from build123d import *

# Parameters (mm, degrees)
F1_DEPTH = 19.05
F2_R     = 88.9
F3_R     = 12.69999
F5_DEPTH = 19.051


# Not quite as in the source:
# - a fillet or chamfer is up to 0.001 mm smaller than in the source, because OpenCascade refuses the exact size


with BuildPart() as f1:
    # F0 (on Front) → F1 (new body)
    with BuildSketch(Plane.XZ):
        Polygon((0, 241.3), (0, 0), (43.18, 0), (43.18, 101.6), (144.78, 101.6), (144.78, 139.7), (43.18, 139.7), (43.18, 241.3), align=None)
    extrude(amount=F1_DEPTH)

    # F2
    f2_edges = [f1.edges().sort_by_distance(p)[0] for p in [
        (43.18, -9.525, 101.6),
    ]]
    fillet(f2_edges, radius=F2_R)

    # F3 (radius 12.7 in the source; OpenCascade refuses exactly that, so slightly less here)
    f3_edges = [f1.edges().sort_by_distance(p)[0] for p in [
        (144.78, -9.525, 139.7),
        (144.78, -9.525, 101.6),
        (43.18, -9.525, 0),
        (43.18, -9.525, 241.3),
        (0, -9.525, 0),
        (0, -9.525, 241.3),
    ]]
    fillet(f3_edges, radius=F3_R)

    # F4 (on face) → F5 (cut, through all)
    with BuildSketch(Plane.XZ.offset(19.05)):
        with BuildLine():
            Line((43.18, 139.7), (43.18, 147.32))
            ThreePointArc((43.18, 147.32), (39.37, 143.51), (43.18, 139.7))
        make_face()
    extrude(amount=-F5_DEPTH, mode=Mode.SUBTRACT)


solid = f1.part
The listing builds one solid part. Answer for the finished solid, in the listing's coordinates (mm). A direction names the side the tool comes from. Round coordinates to 2 decimals unless told otherwise and drop trailing zeros. Write each loop counter-clockwise with the first axis right and the second up, starting at its lowest first coordinate (ties: lowest second). Pieces come first, ordered by that corner, then holes. Notation, with made-up numbers: (63, 4) - (109, 4) arc R5 cw to (109, 10) - close; hole circle Ø1 at (18.25, 75). An arc over 180 degrees is marked (long way). Use a Markdown table: item, result. Add a question column.
1. A tool of negligible diameter and unlimited length cuts with its end or side. For faces 4 (the face through (140.96, -9.66, 105.22)), 5 (the face through (88, -9, 139.7)), from which of +Z, -Z, +X, -X, +Y, -Y can it reach the whole face along a straight path? Write none if from no direction.
2. Consider line 1 (Z direction, x = 133, y = -8.5); line 2 (X direction, y = -9, z = 218); line 3 (Z direction, x = 6.5, y = -13.75). Determine where each line is inside the solid, lowest interval first.
3. For a pull along Z with two mould halves and no side action, classify faces 1 (the face through (39.36, -9.66, 237.68)), 2 (the face through (3.82, -9.66, 3.62)), 3 (the face through (39.37, -9.66, 143.59)) as +Z half, -Z half, draft (parallel to the pull), parting line (faces both ways), or undercut.
4. The part is cut by section B-B (z = 179.5). Write down the section's boundary in (x, y).
5. Flat-ended cylindrical pins translate along their axes: P1, Ø3, axis at x = 86, z = 93.5, coming from the +Y side; P2, Ø9.5, axis at x = 69.5, y = -14, coming from the +Z side; P3, Ø1.5, axis at y = -14.5, z = 77.5, coming from the +X side. Find the tip coordinate at first contact, or state that the pin passes through.
6. The part is cut by section C-C (x = 58). Write down the section's boundary in (y, z).
Reported:
| question | item | result |
|---|---|---|
| 1 | face 4 | -Z, +X, +Y, -Y |
| 1 | face 5 | +Z, +X, +Y, -Y |
| 2 | line 1 | 101.63 to 139.67 |
| 2 | line 2 | 0 to 43.18 |
| 2 | line 3 | 1.62 to 239.68 |
| 3 | face 1 | +Z half |
| 3 | face 2 | -Z half |
| 3 | face 3 | undercut |
| 4 | outline | (0, -19.05) - (43.18, -19.05) - (43.18, 0) - (0, 0) - close |
| 5 | P1 | y = 0 |
| 5 | P2 | z = 139.7 |
| 5 | P3 | x = 72.03 |
| 6 | outline | (-19.05, 61.85) - (0, 61.85) - (0, 139.7) - (-19.05, 139.7) - close |
